Part model, mm, in its own coordinate system. Round coordinates to 2 decimals unless told otherwise and drop trailing zeros. Write each loop counter-clockwise with the first axis right and the second up, starting at its lowest first coordinate (ties: lowest second). Pieces come first, ordered by that corner, then holes. Notation, with made-up numbers: M 56,-37 L 93,-37 A24 cw 93,-26 Z; hole C 0,-8 d11. An arc over 180 degrees is marked long. Answer as a JSON object with one key per item and string values. Group by question number.
1. Band-saw the part on C-C, the plane z = 10. Write the cut outline in (x, y).
2. Drill centre lines: line 1 (Z direction, x = 10, y = 3); line 2 (Z direction, x = -20, y = 4); line 3 (X direction, y = 0.75, z = 20.5). Where is each one in solid material? Low to high. Write a range as from..to.
3. Band-saw the part on B-B, the plane y = 4.5. Count the separate pieces of the cut face and the enclosed holes in it, plus the area to 3 significant figures.
4. Drop flat-ended pins along their axis: pin 1 (3 mm diameter, centred on x = -10, z = -10, fed in from -Y); pin 2 (4 mm diameter, centred on x = 10, z = -10, fed in from -Y). Give the stop position or say it passes through.
5. Band-saw the part on A-A, the plane x = -20. Write the cut outline in (y, z), plus the area to 3 significant figures.
Autodesk Inventor part; units mm, degrees
ref_plane "YZ Plane" through (0, 0, 0) normal (1, 0, 0) x (0, 1, 0)
ref_plane "XZ Plane" through (0, 0, 0) normal (0, 1, 0) x (-1, 0, 0)
ref_plane "XY Plane" through (0, 0, 0) normal (0, 0, 1) x (1, 0, 0)
sketch "Sketch2" plane through (0, 0, 0) normal (0, 1, 0) x (-1, 0, 0)
  line L0 (-10, 10) -> (10, 10) construction
  line L1 (10, 10) -> (10, -10) construction
  line L2 (10, -10) -> (-10, -10) construction
  line L3 (-10, -10) -> (-10, 10) construction
  line L4 (-10, 10) -> (10, -10) construction
  line L5 (10, 10) -> (-10, -10) construction
  line L6 (-20, 20) -> (20, 20) construction
  line L7 (20, 20) -> (20, -20) construction
  line L8 (20, -20) -> (-20, -20) construction
  line L9 (-20, -20) -> (-20, 20) construction
  line L10 (-20, 20) -> (20, -20) construction
  line L11 (20, 20) -> (-20, -20) construction
  line L12 (-30, 25) -> (30, 25)
  line L13 (30, 25) -> (30, -25)
  line L14 (30, -25) -> (-30, -25)
  line L15 (-30, -25) -> (-30, 25)
  line L16 (-30, 25) -> (30, -25) construction
  line L17 (30, 25) -> (-30, -25) construction
  circle A0 centre (-20, -20) radius 2.6
  circle A1 centre (20, -20) radius 2.6
  circle A2 centre (20, 20) radius 2.6
  circle A3 centre (-20, 20) radius 2.6
  circle A4 centre (-10, -10) radius 1.6
  circle A5 centre (10, -10) radius 1.6
  circle A6 centre (10, 10) radius 1.6
  circle A7 centre (-10, 10) radius 1.6
  point P0 (0, 0)
  dimension "d7" = 40
  dimension "d8" = 60
  dimension "d9" = 20
  dimension "d10" = 5.2
  dimension "d11" = 3.2
  dimension "d17" = 50
extrude "Extrusion2" add sketch "Sketch2" along normal blind 7
sketch "Sketch3" plane through (-30, 0, 25) normal (0, 0, 1) x (1, 0, 0)
  circle A0 centre (30, 3.5) radius 1.6
  line L0 (0, 0) -> (60, 0)
  line L1 (60, 0) -> (60, 7)
  point P0 (30, 0)
  point P1 (30, 0)
  point P2 (60, 3.5)
  dimension "d14" = 3.2
extrude "Extrusion3" [suppressed]
properties part number "Master"
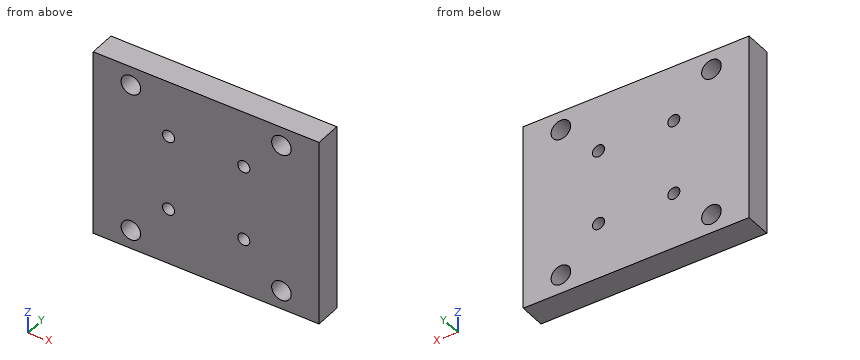
Worked answers:
{
 "1": {"outline": "M -30,0 L -11.6,0 L -11.6,7 L -30,7 Z; M -8.4,0 L 8.4,0 L 8.4,7 L -8.4,7 Z; M 11.6,0 L 30,0 L 30,7 L 11.6,7 Z"},
 "2": {"line 1": "z = -25..-11.6, -8.4..8.4, 11.6..25", "line 2": "z = -25..-22.6, -17.4..17.4, 22.6..25", "line 3": "x = -30..-22.55, -17.45..17.45, 22.55..30"},
 "3": {"separate pieces": "1", "enclosed holes": "8", "area": "2,880 mm^2"},
 "4": {"pin 1": "passes through", "pin 2": "stops at y = 0"},
 "5": {"outline": "M 0,-25 L 7,-25 L 7,-22.6 L 0,-22.6 Z; M 0,-17.4 L 7,-17.4 L 7,17.4 L 0,17.4 Z; M 0,22.6 L 7,22.6 L 7,25 L 0,25 Z", "area": "277 mm^2"}
}
